from build123d import *

# Parameters (mm, degrees)
F2_R      = 9.751517
F3_DEPTH  = 21.591
F3_FACE_R = 9.751517
F4_DEPTH  = 21.591


with BuildPart() as f1:
    # F0 (on Front) → F1 (revolve)
    with BuildSketch(Plane.XZ):
        with BuildLine():
            Line((-10.593969, 33.663088), (-10.593969, -23.486912))
            Line((-10.593969, -23.486912), (10.996031, -23.486912))
            Line((10.996031, -23.486912), (10.996031, 42.807088))
            ThreePointArc((10.996031, 42.807088), (-0.727246, 40.426852), (-10.593969, 33.663088))
        make_face()
    revolve(axis=Axis((10.996031, 0, 9.660088), (0, 0, -1)))

    # F2 (on Front) → F3 (cut, through all)
    with BuildSketch(Plane.XZ):
        with Locations((10.654598, 15.278292)):
            Circle(F2_R)
    extrude(amount=-F3_DEPTH, mode=Mode.SUBTRACT)

    # F3_face (on face) → F4 (cut, through all)
    with BuildSketch(Plane(origin=(10.654598, 0, 15.278292), x_dir=(1, 0, 0), z_dir=(0, 1, 0))):
        Circle(F3_FACE_R)
    extrude(amount=-F4_DEPTH, mode=Mode.SUBTRACT)


solid = f1.part
Verification items for the finished model (mm, model axes). Give positions to 0.01 mm unless a question says otherwise; leave off trailing zeros. Order: outer loops, then holes, each group sorted by start corner. A loop starts at its lowest first (then second) coordinate and runs counter-clockwise, first axis right, second up. Notation, with made-up numbers: M 15.25,69.5 L 33.25,69.5 A15 ccw 33.25,88.5 Z; hole C -9,-35 d3. An arc over 180 degrees is marked long. Use one line per item in the form item = value. Start each with the question number.
Q1. Mould release check, pull along X, two halves, no side actions. Record for faces 1 (the cylindrical face through (1.03, -19.15, 4.69)), 2 (the flat face through (11, 0, -23.487)), 3 (the cylindrical face through (19.663, 0.302, 19.013)): +X half, -X half, draft (parallel to the pull), parting line (faces both ways), or undercut.
Q2. Go/stop test with flat-tipped pins: pin 1 Ø10 at (y, z) = (17, 18) entering from -X; pin 2 Ø4 at (y, z) = (11, -8) entering from +X; pin 3 Ø8 at (y, z) = (-2.5, -2.5) entering from +X; pin 4 Ø8 at (x, z) = (-5.5, -15) entering from +Y. Record where each tip stops, or that it passes through.
Q3. Section check A-A (z = 28.5). Enter the section's corners in (x, y).
Q4. Section check B-B (z = 14.5). Enter the section's corners in (x, y) (3 decimals).
Q5. Scan lines: line 1 along Z through (x, y) = (5.5, 0); line 2 along Z through (x, y) = (7, -17); line 3 along X through (y, z) = (16.5, 6.5). Record each from-to range of solid material in increasing order. Write a range as [from, to].
Evaluation:
q1.face_1 = parting line
q1.face_2 = draft
q1.face_3 = undercut
q2.pin_1 = -6.95
q2.pin_2 = 30.62
q2.pin_3 = 32.59
q2.pin_4 = 17.61
q3.outline = C 11,0 d43.18
q4.outline = M 0.934,-19.102 L 0.934,19.102 A21.59 ccw Z; M 20.375,-19.446 A21.59 ccw 20.375,19.446 Z
q5.line_1 = [-23.49, 7], [23.56, 42.3]
q5.line_2 = [-23.49, 6.24], [24.32, 37.21]
q5.line_3 = [-2.93, 6.41], [14.9, 24.92]
